from build123d import *

# Parameters (mm, degrees)
F0_W         = 105.2784845233
F0_H         = 83.1132326275
F1_DEPTH     = 15.24
F2_SIZE      = 5.08
F3_SIZE      = 5.08
F4_R         = 17.3387510066
F4_R_2       = 5.4081350991
F5_DEPTH     = 2.54
F6_W         = 68.5574207455
F6_H         = 7.6610487886
F7_DEPTH     = 0.254
F8_W         = 72.6598203182
F8_H         = 7.5589888729
F9_DEPTH     = 0.254
F10_T1_DEPTH = 13.3181495789
F11_R        = 5.08
F12_T1_DEPTH = 13.3181495789
F13_R        = 5.08


# Not quite as in the source:
# - a fillet or chamfer that OpenCascade refuses, or shapes differently, is made with other operations: its cross-section is extruded or revolved along the edge and cut away or added


with BuildPart() as f1:
    # F0 (on Top) → F1 (new body)
    with BuildSketch(Plane.XY):
        with Locations((16.9621892273, -13.4625034407)):
            Rectangle(F0_W, F0_H)
    extrude(amount=F1_DEPTH)

    # F2
    f2_edges = [f1.edges().sort_by_distance(p)[0] for p in [
        (-35.677053, -13.462503, 15.24),
        (-35.677053, -13.462503, 0),
    ]]
    chamfer(f2_edges, length=F2_SIZE)

    # F3
    f3_edges = [f1.edges().sort_by_distance(p)[0] for p in [
        (69.601431, -13.462503, 0),
    ]]
    chamfer(f3_edges, length=F3_SIZE)

    # F4 (on face) → F5 (join)
    with BuildSketch(Plane.XY.offset(15.24)):
        with Locations((14.2443789936, 0)):
            Circle(F4_R)
        with Locations((-15.9631352872, -34.4845345244)):
            Circle(F4_R_2)
    extrude(amount=F5_DEPTH)

    # F6 (on face) → F7 (join)
    with BuildSketch(Plane(origin=(0, 28.0941128731, 0), x_dir=(-1, 0, 0), z_dir=(0, 1, 0))):
        with Locations((-17.0010654256, 7.0315066259)):
            Rectangle(F6_W, F6_H)
    extrude(amount=F7_DEPTH)

    # F8 (on face) → F9 (join)
    with BuildSketch(Plane.XZ.offset(55.0191197544)):
        with Locations((14.8761942983, 7.3211907875)):
            Rectangle(F8_W, F8_H)
    extrude(amount=F9_DEPTH)

    # F10: chamfer of 5.08 on 4 edges, made by hand

    # F10_s2 → F10_t1 (cut)
    with BuildSketch(Plane.XZ.offset(55.0191197544)):
        Polygon((51.2061044574, 8.621696351), (46.1261044574, 3.541696351), (51.2061044574, 3.541696351), align=None)
        Polygon((51.2061044574, 6.0206852239), (46.1261044574, 11.1006852239), (51.2061044574, 11.1006852239), align=None)
        Polygon((-21.4537158608, 6.0206852239), (-16.3737158608, 11.1006852239), (-21.4537158608, 11.1006852239), align=None)
        Polygon((-16.3737158608, 3.541696351), (-21.4537158608, 8.621696351), (-21.4537158608, 3.541696351), align=None)
    extrude(amount=F10_T1_DEPTH, mode=Mode.SUBTRACT)

    # F11
    f11_edges = [f1.edges().sort_by_distance(p)[0] for p in [
        (-20.15321, -55.14612, 7.321191),
        (49.905599, -55.14612, 7.321191),
    ]]
    fillet(f11_edges, radius=F11_R)

    # F12: chamfer of 5.08 on 4 edges, made by hand

    # F12_s2 → F12_t1 (cut)
    with BuildSketch(Plane.XZ.offset(-41.4122624519)):
        Polygon((51.2797757983, 5.7820310202), (46.1997757983, 10.8620310202), (51.2797757983, 10.8620310202), align=None)
        Polygon((46.1997757983, 3.2009822316), (51.2797757983, 8.2809822316), (51.2797757983, 3.2009822316), align=None)
        Polygon((-17.2776449472, 8.2809822316), (-12.1976449472, 3.2009822316), (-17.2776449472, 3.2009822316), align=None)
        Polygon((-17.2776449472, 5.7820310202), (-12.1976449472, 10.8620310202), (-17.2776449472, 10.8620310202), align=None)
    extrude(amount=F12_T1_DEPTH, mode=Mode.SUBTRACT)

    # F13
    f13_edges = [f1.edges().sort_by_distance(p)[0] for p in [
        (-16.028169, 28.221113, 7.031507),
        (50.0303, 28.221113, 7.031507),
    ]]
    fillet(f13_edges, radius=F13_R)


solid = f1.part
Verification items for the finished model (mm, model axes). A direction names the side the tool comes from. Give positions to 0.01 mm unless a question says otherwise; leave off trailing zeros. Loops run counter-clockwise (first coordinate to the right, second up) from the corner with the lowest first, then second, coordinate; pieces in that order, holes last. Notation, with made-up numbers: (-3, -35.75) - (5, -35.75) arc R17 cw to (5, -21.75) - close; hole circle Ø9 at (-38.5, 23.25). An arc over 180 degrees is marked (long way). Write item = value, one per line. Start each with the question number.
Q1. Tool access check on faces 5 (the face through (16, 28.094, 13)), 6 (the face through (19, -22, 15.24)), 7 (the face through (69.601, -14, 10)). Record the directions out of +Z, -Z, +X, -X, +Y, -Y that give a thin tool (end or side, any length) a straight path to the whole face; none if there is none.
Q2. Thickness scan on line 1 (Z direction, x = 3, y = -15); line 2 (Y direction, x = 57, z = 1.5); line 3 (X direction, y = -38, z = 1.75). Record the ranges inside material, lowest first.
Q3. Depth check by flat-ended pin: P1, Ø4, axis at x = 49.5, y = -26, coming from the +Z side; P2, Ø1.5, axis at y = 14, z = 2.5, coming from the +X side; P3, Ø3, axis at y = 16, z = 2, coming from the +X side. Enter the tip coordinate at first touch or a pass-through.
Q4. Mould release check, pull along Y, two halves, no side actions. Record for faces 1 (the face through (16, -55.019, 13)), 2 (the face through (17, 28.348, 7)), 3 (the face through (-33.101, -14.044, 2.504)), 4 (the face through (-16.667, -29.122, 16.492)): released by +Y, released by -Y, zero draft, split by the parting line, or undercut.
Q5. Cross-section at C-C, the plane y = 21. Enter the section's corners in (x, z).
Q6. Cross-section at B-B, the plane x = 63. Enter the section's corners in (y, z), and give its area (3 significant figures).
Q7. Cross-section at A-A, the plane y = 0. Enter the section's corners in (x, z).
Q8. Cross-section at D-D, the plane z = 12.75. Enter the section's corners in (x, y), and give its area (3 significant figures).
Answer key:
q1.face_5 = +Y
q1.face_6 = +Z
q1.face_7 = +Z, -Z, +X, +Y, -Y
q2.line_1 = 0 to 15.24
q2.line_2 = -55.02 to 28.09
q2.line_3 = -32.35 to 66.27
q3.P1 = 15.24
q3.P2 = 67.77
q3.P3 = 68.02
q4.face_1 = released by -Y
q4.face_2 = released by +Y
q4.face_3 = zero draft
q4.face_4 = split by the parting line
q5.outline = (-35.68, 5.08) - (-30.6, 0) - (64.52, 0) - (69.6, 5.08) - (69.6, 15.24) - (-30.6, 15.24) - (-35.68, 10.16) - close
q6.outline = (-55.02, 0) - (28.09, 0) - (28.09, 15.24) - (-55.02, 15.24) - close
q6.area = 1,270 mm^2
q7.outline = (-35.68, 5.08) - (-30.6, 0) - (64.52, 0) - (69.6, 5.08) - (69.6, 15.24) - (31.58, 15.24) - (31.58, 17.78) - (-3.09, 17.78) - (-3.09, 15.24) - (-30.6, 15.24) - (-35.68, 10.16) - close
q8.outline = (-33.09, -55.02) - (69.6, -55.02) - (69.6, 28.09) - (-33.09, 28.09) - close
q8.area = 8,530 mm^2
